For this review, take the finished solid that the model builds, in its own axes (mm). Coordinates: 2 decimals unless noted, no trailing zeros. Write each loop counter-clockwise with the first axis right and the second up, starting at its lowest first coordinate (ties: lowest second). Pieces come first, ordered by that corner, then holes.
1) We need section C-C on z = -115. Write out the cut boundary in (x, y).
2) Insertion check: P1, Ø10, axis at x = 33.5, y = 34.5, coming from the -Z side; P2, Ø3, axis at x = 16.5, y = 86, coming from the +Z side; P3, Ø4, axis at x = 28.5, y = 131.5, coming from the +Z side. Each pin has a flat end and moves straight along its axis. Give the tip position at first contact, or say it passes through.
3) We need section A-A on z = -127. Write out the cut boundary in (x, y).
4) To check wall thickness, follow line 1 along Y through (x, z) = (5, -127); line 2 along X through (y, z) = (43, -120.5); line 3 along Z through (x, y) = (6, 17.5) (3 decimals). State the ranges of each line that lie inside material, in increasing order.
5) Mouldability with a two-part tool opening along X and no side actions: class faces 1 (the face through (35.52, 163.19, -143.26)), 2 (the face through (3.302, 81, -130)), 3 (the face through (22.43, 81.394, -144.317)) as pulls with the +X half, pulls with the -X half, needs draft (parallel to the pull), parting line crosses it, or undercut.
from build123d import *

# Parameters (mm, degrees)
BOSS_EXTRUDE1_DEPTH            = 165.1
FILLET1_R                      = 6.35
FILLET2_R                      = 1.5875
SKETCH2_R                      = 3.175
CUT_EXTRUDE1_DEPTH             = 35.385404243
CUT_EXTRUDE2_REACH             = 39.698
SKETCH3_R                      = 3.175
CUT_EXTRUDE2_DIRECTION_2_REACH = 6.755


with BuildPart() as part:
    # Sketch1 → Boss-Extrude1 (new body)
    with BuildSketch(Plane(origin=(0, 0, 0), x_dir=(1, 0, 0), z_dir=(0, 1, 0))):
        with BuildLine():
            ThreePointArc((6.477, 145.90630888), (21.802443449, 144.413489535), (36.88554448, 141.315459552))
            Line((36.88554448, 141.315459552), (37.687404143, 144.38753476))
            ThreePointArc((37.687404143, 144.38753476), (20.634801681, 147.791425951), (3.302, 149.188462761))
            Line((3.302, 149.188462761), (3.302, 146.012668272))
            ThreePointArc((3.302, 146.012668272), (4.889789191, 145.968121388), (6.477, 145.90630888))
        make_face()
        with BuildLine():
            Line((3.302, 146.012668272), (3.302, 111.125))
            Line((3.302, 111.125), (6.477, 111.125))
            Line((6.477, 111.125), (6.477, 145.90630888))
            ThreePointArc((6.477, 145.90630888), (4.889789191, 145.968121388), (3.302, 146.012668272))
        make_face()
    extrude(amount=BOSS_EXTRUDE1_DEPTH)

    # Fillet1
    fillet1_edges = [part.edges().sort_by_distance(p)[0] for p in [
        (37.286474311, 165.1, -142.851497156),
        (4.8895, 165.1, -111.125),
        (4.8895, 0, -111.125),
        (37.286474311, 0, -142.851497156),
    ]]
    fillet(fillet1_edges, radius=FILLET1_R)

    # Fillet2
    fillet2_edges = [part.edges().sort_by_distance(p)[0] for p in [
        (6.477, 82.55, -145.90630888),
    ]]
    fillet(fillet2_edges, radius=FILLET2_R)

    # Sketch2 → Cut-Extrude1 (cut, through all)
    with BuildSketch(Plane.ZY.offset(-3.302)):
        with Locations((-127, 15.875)):
            Circle(SKETCH2_R)
        with Locations((-127, 149.225)):
            Circle(SKETCH2_R)
    extrude(amount=-CUT_EXTRUDE1_DEPTH, mode=Mode.SUBTRACT)

    # Sketch3 → Cut-Extrude2 (cut, up to next)
    with BuildSketch(Plane(origin=(20.494702071, 0, -146.78799876), x_dir=(-0.990393205, 0, -0.13827979), z_dir=(0.13827979, 0, -0.990393205)), mode=Mode.PRIVATE) as cut_extrude2_sk1:
        with Locations((-1.484470958, 15.875)):
            Circle(SKETCH3_R)
    cut_extrude2_tool1 = extrude(cut_extrude2_sk1.sketch, amount=-CUT_EXTRUDE2_REACH, mode=Mode.PRIVATE) & part.part
    add(cut_extrude2_tool1.solids().sort_by_distance((21.964912, 15.875, -146.582726))[0], mode=Mode.SUBTRACT)
    # Sketch3 → Cut-Extrude2 (cut, up to next)
    with BuildSketch(Plane(origin=(20.494702071, 0, -146.78799876), x_dir=(-0.990393205, 0, -0.13827979), z_dir=(0.13827979, 0, -0.990393205)), mode=Mode.PRIVATE) as cut_extrude2_sk2:
        with Locations((-1.484470958, 149.225)):
            Circle(SKETCH3_R)
    cut_extrude2_tool2 = extrude(cut_extrude2_sk2.sketch, amount=-CUT_EXTRUDE2_REACH, mode=Mode.PRIVATE) & part.part
    add(cut_extrude2_tool2.solids().sort_by_distance((21.964912, 149.225, -146.582726))[0], mode=Mode.SUBTRACT)

    # Sketch3 → Cut-Extrude2 direction 2 (cut, up to next)
    with BuildSketch(Plane(origin=(20.494702071, 0, -146.78799876), x_dir=(-0.990393205, 0, -0.13827979), z_dir=(0.13827979, 0, -0.990393205)), mode=Mode.PRIVATE) as cut_extrude2_direction_2_sk1:
        with Locations((-1.484470958, 15.875)):
            Circle(SKETCH3_R)
    cut_extrude2_direction_2_tool1 = extrude(cut_extrude2_direction_2_sk1.sketch, amount=CUT_EXTRUDE2_DIRECTION_2_REACH, mode=Mode.PRIVATE) & part.part
    add(cut_extrude2_direction_2_tool1.solids().sort_by_distance((21.964912, 15.875, -146.582726))[0], mode=Mode.SUBTRACT)
    # Sketch3 → Cut-Extrude2 direction 2 (cut, up to next)
    with BuildSketch(Plane(origin=(20.494702071, 0, -146.78799876), x_dir=(-0.990393205, 0, -0.13827979), z_dir=(0.13827979, 0, -0.990393205)), mode=Mode.PRIVATE) as cut_extrude2_direction_2_sk2:
        with Locations((-1.484470958, 149.225)):
            Circle(SKETCH3_R)
    cut_extrude2_direction_2_tool2 = extrude(cut_extrude2_direction_2_sk2.sketch, amount=CUT_EXTRUDE2_DIRECTION_2_REACH, mode=Mode.PRIVATE) & part.part
    add(cut_extrude2_direction_2_tool2.solids().sort_by_distance((21.964912, 149.225, -146.582726))[0], mode=Mode.SUBTRACT)


solid = part.part
Result:
1. outline: (3.3, 0.5) - (6.48, 0.5) - (6.48, 164.6) - (3.3, 164.6) - close
2. P1: stops at z = -146.48
2. P2: stops at z = -144.94
2. P3: stops at z = -142.83
3. outline: (3.3, 0) - (6.48, 0) - (6.48, 12.7) - (3.3, 12.7) - close; (3.3, 19.05) - (6.48, 19.05) - (6.48, 146.05) - (3.3, 146.05) - close; (3.3, 152.4) - (6.48, 152.4) - (6.48, 165.1) - (3.3, 165.1) - close
4. line 1: y = 0 to 12.7, 19.05 to 146.05, 152.4 to 165.1
4. line 2: x = 3.3 to 6.48
4. line 3: z = -149.104 to -129.728, -124.272 to -111.125
5. face 1: pulls with the +X half
5. face 2: pulls with the -X half
5. face 3: undercut
